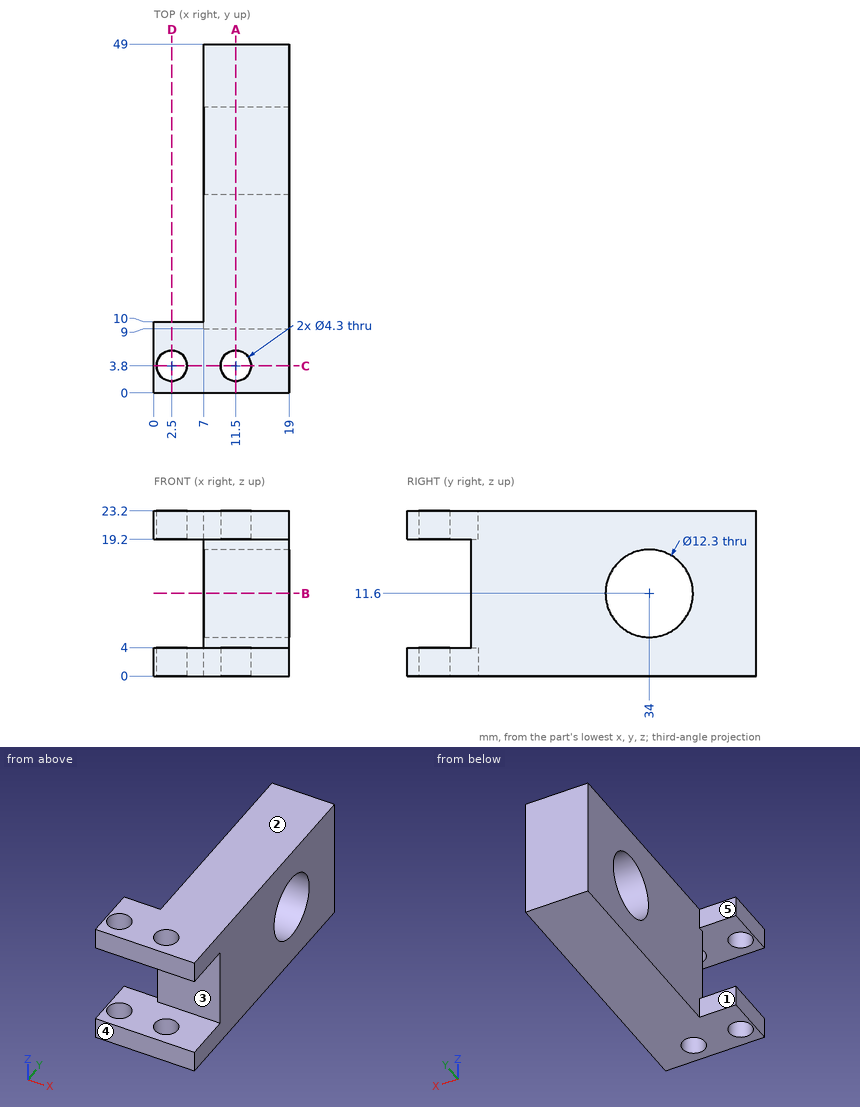
Could you check a few things on this drawing? It's one solid part, dimensions in mm from its lowest x, y, z. A direction names the side the tool comes from. Coordinates: 2 decimals unless noted, no trailing zeros. Loops run counter-clockwise (first coordinate to the right, second up) from the corner with the lowest first, then second, coordinate; pieces in that order, holes last.
1. We'd pull the mould along Z, two halves only. Please class the marked faces 1, 2 and 3: released by +Z, released by -Z, zero draft, split by the parting line, or undercut.
2. I need wall thicknesses on L1, parallel to X at y = 3.8, z = 2.5; L2, parallel to Y at x = 16.75, z = 11.6; L3, parallel to Y at x = 11.5, z = 1.05. Which ranges of each line are inside material? Lowest first, please.
3. Imagine slicing it at A-A (x = 11.5). Please give me the cut outline in (y, z), and give its area (3 significant figures).
4. Imagine slicing it at D-D (x = 2.5). Please give me the cut outline in (y, z).
5. For P1, Ø3, axis at y = 5.5, z = 4.5, coming from the -X side; P2, Ø3.5, axis at x = 11.5, y = 3.8, coming from the +Z side; P3, Ø4.5, axis at x = 2.5, z = 2, coming from the +Y side; P4, Ø1, axis at y = 25.5, z = 14.5, coming from the -X side, each with a flat end and sliding along its axis, tell me the tip position at first contact or that it passes through.
6. Imagine slicing it at C-C (y = 3.8). Please give me the cut outline in (x, z).
7. Imagine slicing it at B-B (z = 11.6). Please give me the cut outline in (x, y).
8. For the marked faces 4 and 5, which set-ups out of +Z, -Z, +X, -X, +Y, -Y let a thin tool reach every point of the face, with its end or its side?
Computed values:
1. face 1: zero draft
1. face 2: released by +Z
1. face 3: undercut
2. L1: x = 0 to 0.35, 4.65 to 9.35, 13.65 to 19
2. L2: y = 9 to 27.85, 40.15 to 49
2. L3: y = 0 to 1.65, 5.95 to 49
3. outline: (0, 0) - (1.65, 0) - (1.65, 4) - (0, 4) - close; (0, 19.2) - (1.65, 19.2) - (1.65, 23.2) - (0, 23.2) - close; (5.95, 0) - (49, 0) - (49, 23.2) - (5.95, 23.2) - (5.95, 19.2) - (9, 19.2) - (9, 4) - (5.95, 4) - close; hole circle Ø12.3 at (34, 11.6)
3. area: 847 mm2
4. outline: (0, 0) - (1.65, 0) - (1.65, 4) - (0, 4) - close; (0, 19.2) - (1.65, 19.2) - (1.65, 23.2) - (0, 23.2) - close; (5.95, 0) - (10, 0) - (10, 4) - (5.95, 4) - close; (5.95, 19.2) - (10, 19.2) - (10, 23.2) - (5.95, 23.2) - close
5. P1: stops at x = 0
5. P2: passes through
5. P3: stops at y = 10
5. P4: stops at x = 7
6. outline: (0, 0) - (0.35, 0) - (0.35, 4) - (0, 4) - close; (0, 19.2) - (0.35, 19.2) - (0.35, 23.2) - (0, 23.2) - close; (4.65, 0) - (9.35, 0) - (9.35, 4) - (4.65, 4) - close; (4.65, 19.2) - (9.35, 19.2) - (9.35, 23.2) - (4.65, 23.2) - close; (13.65, 0) - (19, 0) - (19, 4) - (13.65, 4) - close; (13.65, 19.2) - (19, 19.2) - (19, 23.2) - (13.65, 23.2) - close
7. outline: (7, 9) - (19, 9) - (19, 27.85) - (7, 27.85) - close; (7, 40.15) - (19, 40.15) - (19, 49) - (7, 49) - close
8. face 4: +Z, -Z, +X, -X, -Y
8. face 5: +Z, -Z, -X, +Y
